Geometry: final body of the model. Coordinates: model frame, mm. Face numbers are marked on the shaded views. Give positions to 0.01 mm unless a question says otherwise; leave off trailing zeros. Order: outer loops, then holes, each group sorted by start corner. A loop starts at its lowest first (then second) coordinate and runs counter-clockwise, first axis right, second up. Notation, with made-up numbers: (24.5, -22) - (69.5, -22) arc R16 cw to (69.5, -4) - close; hole circle Ø3 at (76.5, 39.25). An arc over 180 degrees is marked (long way). Use one line per item in the form item = value.
from build123d import *

# Parameters (mm, degrees)
EXTRUDE_1_DEPTH           = 15
CUT_EXTRUDE_1_DEPTH       = 15
SKETCH_5_W                = 3
SKETCH_5_H                = 3
EXTRUDE_2_DEPTH           = 0.68
EXTRUDE_3_DEPTH           = 5
EXTRUDE_3_DEPTH_BACK      = 5
CUT_EXTRUDE_11_DEPTH      = 5
CUT_EXTRUDE_11_DEPTH_BACK = 5
FILLET_1_R                = 0.2
FILLET_5_R                = 0.1


with BuildPart() as part:
    # 草图1 → 凸台-拉伸1 (new body)
    with BuildSketch(Plane.XY):
        Polygon((-5.6, 0), (5.6, 0), (1.762967564, 14.32), (-1.762967564, 14.32), align=None)
    extrude(amount=EXTRUDE_1_DEPTH)

    # 草图2 → 切除-拉伸1 (cut)
    with BuildSketch(Plane.XY.offset(15)):
        with BuildLine():
            Line((-3.681483782, 7.16), (-4.06971235, 5.711111261))
            Line((-4.06971235, 5.711111261), (-3.407492768, 5.533670058))
            ThreePointArc((-3.407492768, 5.533670058), (0.190360002, 6.122701516), (-2.631169509, 8.431483409))
            Line((-2.631169509, 8.431483409), (-3.293255215, 8.608888739))
            Line((-3.293255215, 8.608888739), (-3.681483782, 7.16))
        make_face()
    extrude(amount=-CUT_EXTRUDE_1_DEPTH, mode=Mode.SUBTRACT)

    # 草图5 → 凸台-拉伸2 (add)
    with BuildSketch(Plane(origin=(5.224871131, 1.4, 0), x_dir=(0, 0, -1), z_dir=(0.9659258262890671, 0.2588190451025256, 0))):
        with Locations((-7.5, 5.963190799)):
            Rectangle(SKETCH_5_W, SKETCH_5_H)
    extrude(amount=EXTRUDE_2_DEPTH)

    # 草图6 → 凸台-拉伸3 (add, two sides: drawn at the far end of the back side and taken through both)
    with BuildSketch(Plane(origin=(-1.155158781, 4.311111261, 0), x_dir=(0.965925826289067, 0.2588190451025257, 0), z_dir=(0.2588190451025257, -0.965925826289067, 0)).offset(-EXTRUDE_3_DEPTH_BACK)):
        with BuildLine():
            Line((7.909184627, 5.55), (6.964774906, 5.55))
            ThreePointArc((6.964774906, 5.55), (6.497346154, 5.719957697), (6.086308972, 6))
            Line((6.086308972, 6), (6.086308972, 9))
            ThreePointArc((6.086308972, 9), (6.497346154, 9.280042303), (6.964774906, 9.45))
            Line((6.964774906, 9.45), (7.909184627, 9.45))
            Line((7.909184627, 9.45), (7.909184627, 5.55))
        make_face()
    extrude(amount=EXTRUDE_3_DEPTH + EXTRUDE_3_DEPTH_BACK)

    # 草图7 → 切除-拉伸11 (cut, two sides: drawn at the far end of the back side and taken through both)
    with BuildSketch(Plane.XY.offset(9).offset(-CUT_EXTRUDE_11_DEPTH_BACK)):
        with BuildLine():
            Line((5.59160121, 9.690602974), (4.67937147, 9.446171752))
            ThreePointArc((4.67937147, 9.446171752), (4.271858255, 9.16102576), (3.947307106, 8.784141416))
            Line((3.947307106, 8.784141416), (3.429669016, 10.715993068))
            Line((3.429669016, 10.715993068), (4.27820195, 10.943356783))
            Line((4.27820195, 10.943356783), (5.19043169, 11.187788005))
            Line((5.19043169, 11.187788005), (5.59160121, 9.690602974))
        make_face()
        with BuildLine():
            Line((6.600995486, 5.923492251), (5.688765746, 5.679061029))
            ThreePointArc((5.688765746, 5.679061029), (5.193275954, 5.722248095), (4.723764242, 5.886363937))
            Line((4.723764242, 5.886363937), (6.017859467, 1.056734805))
            Line((6.017859467, 1.056734805), (6.866392401, 1.28409852))
            Line((6.866392401, 1.28409852), (7.778622141, 1.528529742))
            Line((7.778622141, 1.528529742), (6.600995486, 5.923492251))
        make_face()
    extrude(amount=CUT_EXTRUDE_11_DEPTH + CUT_EXTRUDE_11_DEPTH_BACK, mode=Mode.SUBTRACT)

    # 圆角1
    fillet_1_edges = [part.edges().sort_by_distance(p)[0] for p in [
        (0, 0, 15),
        (3.681483782, 7.16, 15),
        (-4.834856175, 2.85555563, 0),
        (-4.834856175, 2.85555563, 15),
        (-3.293255215, 8.608888739, 7.5),
        (-4.06971235, 5.711111261, 7.5),
        (0, 14.32, 15),
        (3.681483782, 7.16, 0),
        (0, 0, 0),
        (-2.528111389, 11.46444437, 0),
        (0, 14.32, 0),
        (-2.528111389, 11.46444437, 15),
        (1.762967564, 14.32, 7.5),
        (5.6, 0, 7.5),
        (-5.6, 0, 7.5),
        (-1.762967564, 14.32, 7.5),
    ]]
    fillet(fillet_1_edges, radius=FILLET_1_R)

    # 圆角5
    fillet_5_edges = [part.edges().sort_by_distance(p)[0] for p in [
        (6.096298348, 7.807047613, 9.45),
        (6.096298348, 7.807047613, 5.55),
        (5.59160121, 9.690602974, 7.5),
        (6.600995486, 5.923492251, 7.5),
    ]]
    fillet(fillet_5_edges, radius=FILLET_5_R)


solid = part.part
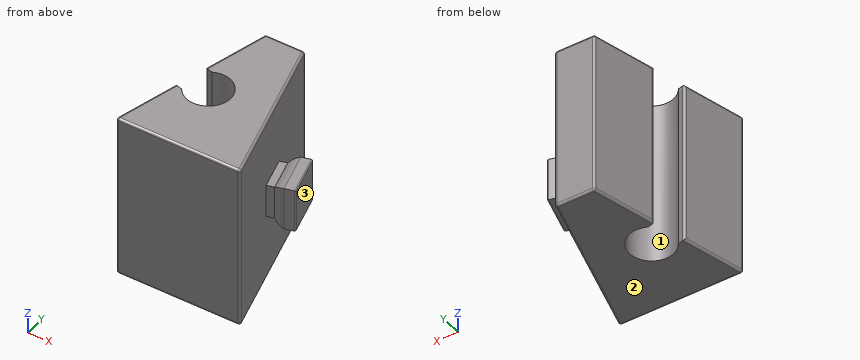
(1) Cut plane A-A on x = 0. Output: boundary loops of the cut face in (y, z), plus the area to 3 significant figures.
Computed values:
outline = (0, 0.2) arc R0.2 ccw to (0.2, 0) - (5.66, 0) - (5.66, 15) - (0.2, 15) arc R0.2 ccw to (0, 14.8) - close; (7.62, 0) - (14.12, 0) arc R0.2 ccw to (14.32, 0.2) - (14.32, 14.8) arc R0.2 ccw to (14.12, 15) - (7.62, 15) - close
area = 185 mm²
(2) Ray query, line 1 along Z through (x, y) = (5.75, 5.75); line 2 along X through (y, z) = (4.5, 0.75); line 3 along X through (y, z) = (9.25, 7.25). Return the intervals inside material, ascending.
Computed values:
line_1 = 5.55 to 9.45
line_2 = -4.39 to 4.39
line_3 = -3.12 to 3.12, 4.38 to 5.71
(3) Contact query for flat-ended pins moving along their axis: pin 1 Ø1.5 at (x, y) = (6, 7) entering from -Z; pin 2 Ø0.9 at (x, y) = (5.5, 7.5) entering from +Z; pin 3 Ø4 at (y, z) = (3.5, 8) entering from -X. Output: stop coordinate, or through.
Computed values:
pin_1 = 5.55
pin_2 = 9.45
pin_3 = -5.2
(4) Cut plane B-B on z = 11. Output: boundary loops of the cut face in (x, y), plus the area to 3 significant figures.
Computed values:
outline = (-5.53, 0.25) arc R0.2 ccw to (-5.34, 0) - (5.34, 0) arc R0.2 ccw to (5.53, 0.25) - (1.8, 14.17) arc R0.2 ccw to (1.61, 14.32) - (-1.61, 14.32) arc R0.2 ccw to (-1.8, 14.17) - (-3.24, 8.8) arc R0.2 ccw to (-3.1, 8.56) - (-2.63, 8.43) arc R2 cw (long way) to (-3.41, 5.53) - (-3.88, 5.66) arc R0.2 ccw to (-4.12, 5.52) - close
area = 92.2 mm²
(5) Pull-direction query (Y, two-part tool) for the marked faces 1, 2 and 3; classes: released by +Y, released by -Y, zero draft, split by the parting line, or undercut.
Computed values:
face_1 = undercut
face_2 = zero draft
face_3 = released by +Y
